Read the model definition and answer for the solid it produces. Units are mm, in the model's axes. A direction names the side the tool comes from. Round coordinates to 2 decimals unless told otherwise and drop trailing zeros. Loops run counter-clockwise (first coordinate to the right, second up) from the corner with the lowest first, then second, coordinate; pieces in that order, holes last. Notation, with made-up numbers: M 58,-12.75 L 77,-12.75 A21 cw 77,6.25 Z; hole C 40,-17.5 d10. An arc over 180 degrees is marked long. Answer as CSV lines item,"result".
```python
from build123d import *

# Parameters (mm, degrees)
SKETCH1_R           = 1.27
BOSS_EXTRUDE1_DEPTH = 4.572
FILLET4_R           = 1.27
FILLET5_R           = 1.27
FILLET6_R           = 8.89
FILLET7_R           = 19.05
FILLET8_R           = 1.016


with BuildPart() as part:
    # Sketch1 → Boss-Extrude1 (new body)
    with BuildSketch(Plane(origin=(0, 0, 0), x_dir=(0, 0, -1), z_dir=(1, 0, 0))):
        Polygon((-5.715, 23.017636755), (-5.715, 4.539136755), (1.905, 4.539136755), (1.905, 10.889136755), (0, 10.889136755), (0, 18.255136755), (1.531272723, 18.255136755), (17.78, 9.623119465), (17.78, 6.545736755), (15.875, 6.545736755), (15.875, -8.732363245), (22.5425, -8.732363245), (22.5425, 23.017636755), align=None)
        with Locations((-0.635, 7.714136755)):
            Circle(SKETCH1_R, mode=Mode.SUBTRACT)
    extrude(amount=BOSS_EXTRUDE1_DEPTH)

    # Fillet4
    fillet4_edges = [part.edges().sort_by_distance(p)[0] for p in [
        (2.286, 4.539136755, 5.715),
        (2.286, 6.545736755, -15.875),
        (2.286, 10.889136755, -1.905),
        (2.286, 4.539136755, -1.905),
    ]]
    fillet(fillet4_edges, radius=FILLET4_R)

    # Fillet5
    fillet5_edges = [part.edges().sort_by_distance(p)[0] for p in [
        (2.286, -8.732363245, -22.5425),
        (2.286, -8.732363245, -15.875),
        (2.286, 9.623119465, -17.78),
        (2.286, 18.255136755, 0),
    ]]
    fillet(fillet5_edges, radius=FILLET5_R)

    # Fillet6
    fillet6_edges = [part.edges().sort_by_distance(p)[0] for p in [
        (2.286, 23.017636755, 5.715),
    ]]
    fillet(fillet6_edges, radius=FILLET6_R)

    # Fillet7
    fillet7_edges = [part.edges().sort_by_distance(p)[0] for p in [
        (2.286, 23.017636755, -22.5425),
    ]]
    fillet(fillet7_edges, radius=FILLET7_R)

    # Fillet8
    fillet8_edges = [part.edges().sort_by_distance(p)[0] for p in [
        (4.572, 13.937136755, 0),
        (0, 6.545736755, -17.4625),
        (0, 14.118204509, -9.318546725),
        (0, 13.937136755, 0),
        (4.572, 14.118204509, -9.318546725),
        (4.572, 6.545736755, -17.4625),
        (0, -1.093313245, -15.875),
        (4.572, -1.093313245, -15.875),
        (0, 4.539136755, 1.905),
        (0, 10.889136755, -0.3175),
        (0, 7.714136755, -1.905),
        (0, 4.911111143, 5.343025612),
        (0, 4.911111143, -1.533025612),
        (0, 10.517162367, -1.533025612),
        (0, 6.173762367, -16.246974388),
        (4.572, 4.539136755, 1.905),
        (4.572, 7.714136755, -1.905),
        (4.572, 10.889136755, -0.3175),
        (4.572, 4.911111143, 5.343025612),
        (4.572, 4.911111143, -1.533025612),
        (4.572, 10.517162367, -1.533025612),
        (4.572, 6.173762367, -16.246974388),
        (0, 18.255136755, -1.400636361),
        (4.572, 18.255136755, -1.400636361),
        (0, 7.702724325, -17.78),
        (4.572, 7.702724325, -17.78),
        (0, -1.747363245, -22.5425),
        (4.572, -1.747363245, -22.5425),
        (0, -8.732363245, -19.20875),
        (0, -8.360388857, -16.246974388),
        (0, -8.360388857, -22.170525612),
        (4.572, -8.732363245, -19.20875),
        (4.572, -8.360388857, -16.246974388),
        (4.572, -8.360388857, -22.170525612),
        (0, 17.883162367, -0.371974388),
        (4.572, 17.883162367, -0.371974388),
        (0, 9.51400834, -17.598483423),
        (4.572, 9.51400834, -17.598483423),
        (0, 9.968386755, 5.715),
        (4.572, 9.968386755, 5.715),
        (0, 20.413816039, 3.111179285),
        (4.572, 20.413816039, 3.111179285),
        (0, 23.017636755, -3.33375),
        (4.572, 23.017636755, -3.33375),
        (0, 17.438020936, -16.962884182),
        (4.572, 17.438020936, -16.962884182),
    ]]
    fillet(fillet8_edges, radius=FILLET8_R)


solid = part.part
```
1) Determine the mould class of faces 6 (the cylindrical face through (4.266, 7.741, -1.615)), 7 (the cylindrical face through (4.266, 22.728, -3.332)), 8 (the flat face through (2, -8.732, -19)), 9 (the cylindrical face through (0.29, 7.541, -18.086)) for opening direction Y: released by +Y, released by -Y, zero draft, split by the parting line, or undercut.
Evaluation:
face 6,"zero draft"
face 7,"released by +Y"
face 8,"released by -Y"
face 9,"undercut"
2) Each of these flat-tipped pins is pushed along its axis until it touches: P1, Ø8, axis at y = 4, z = -7, coming from the -X side; P2, Ø0.8, axis at x = 3, y = 7, coming from the -Z side; P3, Ø0.5, axis at x = 2.5, z = -0.5, coming from the +Y side; P4, Ø1.3, axis at x = 2.5, z = 1.5, coming from the -Y side. Where does it stop, or does it pass through?
Evaluation:
P1,"passes through"
P2,"stops at z = -22.36"
P3,"stops at y = 22.68"
P4,"stops at y = 4.54"
3) Find section C-C, the plane y = 8.5. Count the separate pieces of the cut face and the enclosed holes in it, then the cut area to 3 significant figures.
Evaluation:
separate pieces,"3"
enclosed holes,"0"
area,"43.2 mm^2"
4) Find section B-B, the plane y = -4. Give the vertices of the cut face in (x, z) (1 decimal).
Evaluation:
outline,"M 0,-21.5 A1 ccw 1,-22.5 L 3.6,-22.5 A1 ccw 4.6,-21.5 L 4.6,-16.9 A1 ccw 3.6,-15.9 L 1,-15.9 A1 ccw 0,-16.9 Z"
5) Straight lines are drawn through the part: line 1 (Y direction, x = 2.6, z = -0.5); line 2 (Z direction, x = 2.6, y = 3.5) (1 decimal); line 3 (Z direction, x = 1.7, y = 6) (3 decimals). For each, find the intervals that lie inside material, in ascending order.
Evaluation:
line 1,"y = 4.54 to 7.14, 8.28 to 10.89, 18 to 22.61"
line 2,"z = -22.5 to -15.9"
line 3,"z = -22.434 to -16.102, -1.905 to 5.715"
6) A tool of negligible diameter and unlimited length cuts with its end or side. For faces 1 (the cylindrical face through (4.266, 13.479, 0.29)), 2 (the cylindrical face through (2.3, 4.9, -1.52)), 3 (the cylindrical face through (0.29, 4.845, 1.869)), 4 (the cylindrical face through (0.29, 7.74, -1.6)), 5 (the cylindrical face through (0.177, 6.103, -17.775)), from which of +Z, -Z, +X, -X, +Y, -Y can it reach the whole face along a straight path? Write none if from no direction.
Evaluation:
face 1,"+X"
face 2,"+X, -X, -Y"
face 3,"+Z, -X, -Y"
face 4,"-X, -Y"
face 5,"-X"
